from build123d import *

# Parameters (mm, degrees)
F0_W     = 95.25
F0_H     = 19.05
F1_DEPTH = 12.7
F3_DEPTH = 19.051
F4_W     = 25.6279547439
F4_H     = 12.7
F5_DEPTH = 8.382
F7_DEPTH = 12.701


with BuildPart() as f1:
    # F0 (on Front) → F1 (new body)
    with BuildSketch(Plane.XZ):
        with Locations((47.625, 9.525)):
            Rectangle(F0_W, F0_H)
    extrude(amount=F1_DEPTH)

    # F2 (on face) → F3 (cut, through all)
    with BuildSketch(Plane(origin=(0, 0, 0), x_dir=(1, 0, 0), z_dir=(0, 0, -1))):
        with BuildLine():
            Line((18.4131473885, 10.1599995496), (6.9831433348, 10.1544417125))
            ThreePointArc((6.9831433348, 10.1544417125), (3.1749963967, 6.3425895514), (6.9868485577, 2.5344426133))
            Line((6.9868485577, 2.5344426133), (18.4168526115, 2.5400004504))
            ThreePointArc((18.4168526115, 2.5400004504), (22.2249995496, 6.3518526115), (18.4131473885, 10.1599995496))
        make_face()
        with BuildLine():
            Line((76.835, 2.54), (88.265, 2.54))
            ThreePointArc((88.265, 2.54), (92.075, 6.35), (88.265, 10.16))
            Line((88.265, 10.16), (76.835, 10.16))
            ThreePointArc((76.835, 10.16), (73.025, 6.35), (76.835, 2.54))
        make_face()
    extrude(amount=-F3_DEPTH, mode=Mode.SUBTRACT)

    # F4 (on face) → F5 (join)
    with BuildSketch(Plane.XY.offset(19.05)):
        with Locations((82.4360226281, -6.35)):
            Rectangle(F4_W, F4_H)
        with BuildLine():
            ThreePointArc((76.835, -10.16), (73.025, -6.35), (76.835, -2.54))
            Line((76.835, -2.54), (88.265, -2.54))
            ThreePointArc((88.265, -2.54), (92.075, -6.35), (88.265, -10.16))
            Line((88.265, -10.16), (76.835, -10.16))
        make_face(mode=Mode.SUBTRACT)
    extrude(amount=F5_DEPTH)

    # F6 (on face) → F7 (cut, through all)
    with BuildSketch(Plane.XZ.offset(12.7)):
        with BuildLine():
            ThreePointArc((25.6279547439, 19.05), (47.625, 6.35), (69.6220452561, 19.05))
            Line((69.6220452561, 19.05), (25.6279547439, 19.05))
        make_face()
        with BuildLine():
            Line((69.6220452561, 27.432), (69.6220452561, 19.05))
            ThreePointArc((69.6220452561, 19.05), (71.5092373122, 23.1068982411), (72.6552791834, 27.432))
            Line((72.6552791834, 27.432), (69.6220452561, 27.432))
        make_face()
    extrude(amount=-F7_DEPTH, mode=Mode.SUBTRACT)


solid = f1.part
Work out the finished part from the listing and answer in its coordinate system (mm). A direction names the side the tool comes from. Round coordinates to 2 decimals unless told otherwise and drop trailing zeros. Write each loop counter-clockwise with the first axis right and the second up, starting at its lowest first coordinate (ties: lowest second). Pieces come first, ordered by that corner, then holes.
1) A cutting plane is placed at C-C (x = 82.5). Give the vertices of the cut face in (y, z).
2) A tool of negligible diameter and unlimited length cuts with its end or side. For faces 1 (the flat face through (13, -2, 19.05)), 2 (the flat face through (47, -6, 0)), 3 (the cylindrical face through (73.026, -6.434, 13.524)), from which of +Z, -Z, +X, -X, +Y, -Y can it reach the whole face along a straight path? Write none if from no direction.
3) Straight lines are drawn through the part: line 1 (Y direction, x = 83, z = 22.5); line 2 (X direction, y = -8, z = 6.25); line 3 (Y direction, x = 76.5, z = 7.5). For each, find the intervals that lie inside material, in ascending order.
4) Given pin 1 Ø4 at (x, y) = (63.5, -9) entering from +Z, flat-ended and moving along its own axis, determine where the tip first touches the part or whether it passes through.
5) A cutting plane is placed at D-D (z = 12.5). Give the vertices of the cut face in (x, y) (3 decimals), plus the area to 3 significant figures.
6) A cutting plane is placed at A-A (y = -6.35). Give the vertices of the cut face in (x, z) (3 decimals), plus the area to 3 significant figures.
7) A cutting plane is placed at B-B (z = 2). Give the vertices of the cut face in (x, y) (3 decimals).
Completed:
1. outline: (-12.7, 0) - (-10.16, 0) - (-10.16, 27.43) - (-12.7, 27.43) - close; (-2.54, 0) - (0, 0) - (0, 27.43) - (-2.54, 27.43) - close
2. face 1: +Z, -X, +Y, -Y
2. face 2: -Z, +X, -X, +Y, -Y
2. face 3: +Z, -Z
3. line 1: y = -12.7 to -10.16, -2.54 to 0
3. line 2: x = 0 to 3.55, 21.85 to 73.4, 91.7 to 95.25
3. line 3: y = -12.7 to -10.15, -2.55 to 0
4. pin 1: stops at z = 13.7
5. outline: (0, -12.7) - (31.054, -12.7) - (31.054, 0) - (0, 0) - close; (64.196, -12.7) - (95.25, -12.7) - (95.25, 0) - (64.196, 0) - close; hole (6.983, -10.154) - (18.413, -10.16) arc R3.81 ccw to (18.417, -2.54) - (6.987, -2.534) arc R3.81 ccw to start; hole (76.835, -10.16) - (88.265, -10.16) arc R3.81 ccw to (88.265, -2.54) - (76.835, -2.54) arc R3.81 ccw to start
5. area: 523 mm2
6. outline: (0, 0) - (3.175, 0) - (3.175, 19.05) - (0, 19.05) - close; (22.225, 0) - (73.025, 0) - (73.025, 27.432) - (72.655, 27.432) arc R25.4 cw to (25.628, 19.05) - (22.225, 19.05) - close; (92.075, 0) - (95.25, 0) - (95.25, 27.432) - (92.075, 27.432) - close
6. area: 733 mm2
7. outline: (0, -12.7) - (95.25, -12.7) - (95.25, 0) - (0, 0) - close; hole (6.983, -10.154) - (18.413, -10.16) arc R3.81 ccw to (18.417, -2.54) - (6.987, -2.534) arc R3.81 ccw to start; hole (76.835, -10.16) - (88.265, -10.16) arc R3.81 ccw to (88.265, -2.54) - (76.835, -2.54) arc R3.81 ccw to start
